Geometry check sheet. Reference: the model listing, model coordinates, mm. A direction names the side the tool comes from. Give positions to 0.01 mm unless a question says otherwise; leave off trailing zeros. Write each loop counter-clockwise with the first axis right and the second up, starting at its lowest first coordinate (ties: lowest second). Pieces come first, ordered by that corner, then holes. Notation, with made-up numbers: (-31.75, 85) -> (-19.75, 85) arc R10 cw to (-19.75, 91) -> close; hole circle Ø7 at (38.25, -4.75). An arc over 180 degrees is marked (long way). Write item = value, one per line. Start each with the question number.
1. Depth check by flat-ended pin: P1, Ø0.9, axis at x = 57, y = -53, coming from the +Z side; P2, Ø2.5, axis at x = 52.5, z = -3.5, coming from the -Y side; P3, Ø9.5, axis at y = -5, z = -3, coming from the +X side. Enter the tip coordinate at first touch or a pass-through.
2. Cross-section at C-C, the plane y = -37.5. Record the cut outline in (x, z).
3. Cross-section at B-B, the plane x = 67. Record the cut outline in (y, z), plus the area to 3 significant figures.
4. Thickness scan on line 1 along Z through (x, y) = (2.75, -52); line 2 along Y through (x, z) = (2, -50). Record the ranges inside material, lowest first.
5. Cross-section at A-A, the plane z = -28.5. Record the cut outline in (x, y).
6. Cross-section at D-D, the plane y = -20.5. Record the cut outline in (x, z).
7. Set-up check for faces 4 (the cylindrical face through (42.01, -46.43, -56.4)), 5 (the flat face through (5, -52, -2)), 6 (the cylindrical face through (-11.86, -24.534, -29.021)), 7 (the cylindrical face through (42, -8, -48)), 8 (the cylindrical face through (42.01, -10.57, -0.6)): record each of +Z, -Z, +X, -X, +Y, -Y from which the full face is reachable in a straight line by a thin tool's end or side.
8. Mould release check, pull along Y, two halves, no side actions. Record for faces 1 (the cylindrical face through (2.46, -56.4, -56.43)), 2 (the cylindrical face through (2.465, -5.751, -2.615)), 3 (the flat face through (41, -10, -53)): pulls with the +Y half, pulls with the -Y half, needs draft (parallel to the pull), parting line crosses it, or undercut.
```python
from build123d import *

# Parameters (mm, degrees)
SKETCH1_R            = 2.5
BOSS_EXTRUDE2_DEPTH  = 78
CUT_EXTRUDE1_START   = -73
CUT_EXTRUDE1_DEPTH   = 73
FILLET1_R            = 5
FILLET2_R            = 2
FILLET1_OF_MIRROR3_R = 5
FILLET3_R            = 2
SKETCH5_R            = 19.5
BOSS_EXTRUDE3_DEPTH  = 2
SKETCH6_R            = 4
BOSS_EXTRUDE4_DEPTH  = 20


with BuildPart() as part:
    # Sketch1 → Boss-Extrude2 (new body)
    with BuildSketch(Plane(origin=(0, 0, 0), x_dir=(0, 0, -1), z_dir=(1, 0, 0))):
        with BuildLine():
            Line((2, 0), (55, 0))
            ThreePointArc((55, 0), (56.414213562, -0.585786438), (57, -2))
            Line((57, -2), (57, -55))
            ThreePointArc((57, -55), (56.414213562, -56.414213562), (55, -57))
            Line((55, -57), (2, -57))
            ThreePointArc((2, -57), (0.585786438, -56.414213562), (0, -55))
            Line((0, -55), (0, -2))
            ThreePointArc((0, -2), (0.585786438, -0.585786438), (2, 0))
        make_face()
        with Locations((52, -5)):
            Circle(SKETCH1_R, mode=Mode.SUBTRACT)
        with Locations((52, -52)):
            Circle(SKETCH1_R, mode=Mode.SUBTRACT)
        with Locations(Location((5, -52, 0), (0, 0, 180))):
            Circle(SKETCH1_R, mode=Mode.SUBTRACT)
        with Locations(Location((5, -5, 0), (0, 0, 180))):
            Circle(SKETCH1_R, mode=Mode.SUBTRACT)
    extrude(amount=BOSS_EXTRUDE2_DEPTH)

    # Sketch4 → Cut-Extrude1 (cut)
    with BuildSketch(Plane(origin=(78, 0, 0), x_dir=(0, 0, -1), z_dir=(1, 0, 0)).offset(CUT_EXTRUDE1_START)):
        with BuildLine():
            Line((55, 0), (47, 0))
            Line((47, 0), (47, -10))
            Line((47, -10), (57, -10))
            Line((57, -10), (57, -2))
            ThreePointArc((57, -2), (56.414213562, -0.585786438), (55, 0))
        make_face()
        with BuildLine():
            Line((0, -2), (0, -10))
            Line((0, -10), (10, -10))
            Line((10, -10), (10, 0))
            Line((10, 0), (2, 0))
            ThreePointArc((2, 0), (0.585786438, -0.585786438), (0, -2))
        make_face()
    cut_extrude1 = extrude(amount=CUT_EXTRUDE1_DEPTH, mode=Mode.SUBTRACT)

    # Fillet1
    fillet1_edges = [part.edges().sort_by_distance(p)[0] for p in [
        (41.5, -10, -10),
        (41.5, -10, -47),
    ]]
    fillet(fillet1_edges, radius=FILLET1_R)

    # Fillet2
    fillet2_edges = [part.edges().sort_by_distance(p)[0] for p in [
        (41.5, 0, -10),
        (41.5, -10, 0),
        (41.5, -10, -57),
        (41.5, 0, -47),
    ]]
    fillet(fillet2_edges, radius=FILLET2_R)

    # Mirror3: Cut-Extrude1 across plane
    add(cut_extrude1.mirror(Plane.ZX.offset(-28.5)), mode=Mode.SUBTRACT)

    # Fillet1 of Mirror3
    fillet1_of_mirror3_edges = [part.edges().sort_by_distance(p)[0] for p in [
        (41.5, -47, -10),
        (41.5, -47, -47),
    ]]
    fillet(fillet1_of_mirror3_edges, radius=FILLET1_OF_MIRROR3_R)

    # Fillet3
    fillet3_edges = [part.edges().sort_by_distance(p)[0] for p in [
        (41.5, -47, 0),
        (41.5, -57, -10),
        (41.5, -57, -47),
        (41.5, -47, -57),
    ]]
    fillet(fillet3_edges, radius=FILLET3_R)

    # Sketch5 → Boss-Extrude3 (add)
    with BuildSketch(Plane.ZY):
        with Locations(Location((-28.5, -28.5, 0), (0, 0, 180))):
            Circle(SKETCH5_R)
    extrude(amount=BOSS_EXTRUDE3_DEPTH)

    # Sketch6 → Boss-Extrude4 (add)
    with BuildSketch(Plane.ZY.offset(2)):
        with Locations((-28.5, -28.5)):
            Circle(SKETCH6_R)
    extrude(amount=BOSS_EXTRUDE4_DEPTH)


solid = part.part
```
Answers:
q1.P1 = -10
q1.P2 = -47
q1.P3 = 5
q2.outline = (-2, -45.8) -> (0, -45.8) -> (0, -57) -> (78, -57) -> (78, 0) -> (0, 0) -> (0, -11.2) -> (-2, -11.2) -> close
q3.outline = (-57, -45) arc R2 ccw to (-55, -47) -> (-52, -47) arc R5 cw to (-47, -52) -> (-47, -55) arc R2 ccw to (-45, -57) -> (-12, -57) arc R2 ccw to (-10, -55) -> (-10, -52) arc R5 cw to (-5, -47) -> (-2, -47) arc R2 ccw to (0, -45) -> (0, -12) arc R2 ccw to (-2, -10) -> (-5, -10) arc R5 cw to (-10, -5) -> (-10, -2) arc R2 ccw to (-12, 0) -> (-45, 0) arc R2 ccw to (-47, -2) -> (-47, -5) arc R5 cw to (-52, -10) -> (-55, -10) arc R2 ccw to (-57, -12) -> close
q3.area = 2,860 mm^2
q4.line_1 = -57 to -54.5, -49.5 to -7.5, -2.5 to 0
q4.line_2 = -57 to -53.5, -50.5 to -6.5, -3.5 to 0
q5.outline = (-22, -32.5) -> (-2, -32.5) -> (-2, -48) -> (0, -48) -> (0, -57) -> (78, -57) -> (78, 0) -> (0, 0) -> (0, -9) -> (-2, -9) -> (-2, -24.5) -> (-22, -24.5) -> close
q6.outline = (-2, -46.28) -> (0, -46.28) -> (0, -57) -> (78, -57) -> (78, 0) -> (0, 0) -> (0, -10.72) -> (-2, -10.72) -> close
q7.face_4 = -Z, +X, -Y
q7.face_5 = +Z, +X, -Y
q7.face_6 = -X
q7.face_7 = -Z, +X, +Y
q7.face_8 = +Z, +X, +Y
q8.face_1 = pulls with the -Y half
q8.face_2 = undercut
q8.face_3 = pulls with the +Y half
